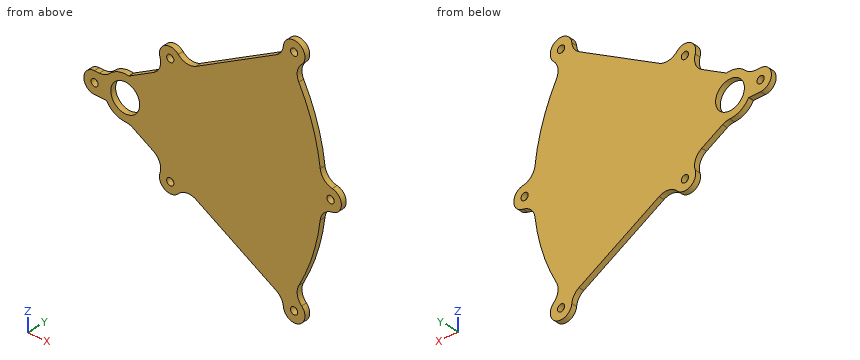
Autodesk Inventor part; units mm, degrees
ref_plane "YZ Plane" through (0, 0, 0) normal (1, 0, 0) x (0, 1, 0)
ref_plane "XZ Plane" through (0, 0, 0) normal (0, 1, 0) x (-1, 0, 0)
ref_plane "XY Plane" through (0, 0, 0) normal (0, 0, 1) x (1, 0, 0)
sketch "Sketch1" plane through (0, 0, 0) normal (0, 1, 0) x (-1, 0, 0)
  circle A0 centre (0, 0) radius 8
  arc A1 (-82.4777, 58.296) -> (-82.4777, -58.296) centre (0, 0) ccw construction
  arc A2 (-86.8253, 60.806) -> (-86.8253, -60.806) centre (0, 0) ccw construction
  arc A3 (-2, -11.8322) -> (-2, 11.8322) centre (0, 0) ccw
  line L0 (-2, -11.8322) -> (-89.433, -62.3116)
  arc A4 (-89.433, 62.3116) -> (-89.433, -62.3116) centre (0, 0) ccw
  line L1 (-2, 11.8322) -> (-89.433, 62.3116)
  circle A5 centre (-93.7631, -64.8116) radius 2
  circle A6 centre (-93.7631, 64.8116) radius 2
  circle A7 centre (-114, 0) radius 2
  circle A8 centre (-25, -30.8847) radius 2
  circle A9 centre (-25, 30.8847) radius 2
  circle A10 centre (17, 0) radius 2
  line L2 (10.3923, -6) -> (17, -6)
  arc A11 (17, -6) -> (17, 6) centre (17, 0) ccw
  line L3 (17, 6) -> (10.3923, 6)
  line L4 (-22.3038, -23.5546) -> (-19.8038, -27.8847)
  arc A12 (-30.1962, -33.8847) -> (-19.8038, -27.8847) centre (-25, -30.8847) ccw
  line L5 (-30.1962, -33.8847) -> (-32.6962, -29.5546)
  line L6 (-22.3038, 23.5546) -> (-19.8038, 27.8847)
  arc A13 (-19.8038, 27.8847) -> (-30.1962, 33.8847) centre (-25, 30.8847) ccw
  line L7 (-30.1962, 33.8847) -> (-32.6962, 29.5546)
  line L8 (-92.8025, 57.1726) -> (-96.9102, 59.7032)
  arc A14 (-88.567, 61.8116) -> (-96.9102, 59.7032) centre (-93.7631, 64.8116) ccw
  line L9 (-108.8347, -6) -> (-114, -6)
  arc A15 (-114, 6) -> (-114, -6) centre (-114, 0) ccw
  line L10 (-114, 6) -> (-108.8347, 6)
  line L11 (-92.8025, -57.1726) -> (-96.9102, -59.7032)
  arc A16 (-96.9102, -59.7032) -> (-88.567, -61.8116) centre (-93.7631, -64.8116) ccw
  point P0 (-109, 0)
  point P1 (12, 0)
  dimension "d0" = 16
  dimension "d1" = 101
  dimension "d3" = 12
  dimension "d6" = 60
  dimension "d7" = 2
  dimension "d8" = 5
  dimension "d9" = 3
  dimension "d10" = 4
  dimension "d12" = 5
  dimension "d13" = 5
  dimension "d14" = 5
  dimension "d15" = 5
  dimension "d16" = 5
  dimension "d17" = 5
  dimension "d18" = 25
  dimension "d19" = 6
  dimension "d20" = 6
extrude "Extrusion1" add sketch "Sketch1" along normal blind 3 contours L0 A4 L1 A3
extrude "Extrusion2" add sketch "Sketch1" along normal blind 3 contours A3 L3 A11 L2 | L4 A12 L5 L0 | A16 L11 A4 L0 | L1 L7 A13 L6 | L1 A4 L8 A14 | L9 A15 L10 A4
fillet "Fillet1" radius 8 12 edges at (32.6962, 1.5, 29.5546) (22.3038, 1.5, 23.5546) (88.567, 1.5, 61.8116) (92.8025, 1.5, 57.1726) (108.8347, 1.5, -6) (108.8347, 1.5, 6) (92.8025, 1.5, -57.1726) (88.567, 1.5, -61.8116) (32.6962, 1.5, -29.5546) (22.3038, 1.5, -23.5546) (2, 1.5, -11.8322) (-10.3923, 1.5, 6)
properties part number "RailBase" material "Polycarbonate, Clear"
Input: part model. Units: mm. Frame: model coordinates. Give positions to 0.01 mm unless a question says otherwise; leave off trailing zeros. Order: outer loops, then holes, each group sorted by start corner. A loop starts at its lowest first (then second) coordinate and runs counter-clockwise, first axis right, second up. Notation, with made-up numbers: (69, 63.5) - (126, 63.5) arc R35 cw to (126, 101.5) - close; hole circle Ø11 at (9, 86.5). An arc over 180 degrees is marked (long way). Answer as a JSON object with one key per item and string values. Group by question number.
Q1. Cut plane A-A, the plane z = 0. Output: boundary loops of the cut face in (x, y), then the cut area to 3 significant figures.
Q2. Line query: probe 1 along Z at (x, y) = (0, 2.1); probe 2 along X at (y, z) = (2.7, 1.5); probe 3 along Z at (x, y) = (-17, 2). Output: solid intervals per line, ascending.
Q3. Cut plane C-C, the plane x = -2. Output: boundary loops of the cut face in (y, z).
Q4. First-contact query: pin 1 Ø3.5 at (x, z) = (-17, 0) entering from +Y; pin 2 Ø1 at (x, z) = (69.5, -27.5) entering from -Y. Flat tips, straight axial feed; report the tip coordinate or a pass-through.
Q5. Cut plane D-D, the plane y = 1.95. Count the separate pieces of the cut face and the enclosed holes in it, then the cut area to 3 significant figures.
Q6. Cut plane B-B, the plane x = 25. Output: boundary loops of the cut face in (y, z).
Results:
{
 "1": {"outline": "(-23, 0) - (-19, 0) - (-19, 3) - (-23, 3) - close; (-15, 0) - (-8, 0) - (-8, 3) - (-15, 3) - close; (8, 0) - (112, 0) - (112, 3) - (8, 3) - close; (116, 0) - (120, 0) - (120, 3) - (116, 3) - close", "area": "357 mm^2"},
 "2": {"probe 1": "-12 to -8, 8 to 12", "probe 2": "-22.81 to -18.32, -15.68 to -7.86, 7.86 to 112.68, 115.32 to 119.81", "probe 3": "-6 to -2, 2 to 6"},
 "3": {"outline": "(0, -11.83) - (3, -11.83) - (3, -7.75) - (0, -7.75) - close; (0, 7.75) - (3, 7.75) - (3, 11.83) - (0, 11.83) - close"},
 "4": {"pin 1": "through", "pin 2": "y = 0"},
 "5": {"separate pieces": "1", "enclosed holes": "7", "area": "8,940 mm^2"},
 "6": {"outline": "(0, -36.88) - (3, -36.88) - (3, -32.88) - (0, -32.88) - close; (0, -28.88) - (3, -28.88) - (3, 28.88) - (0, 28.88) - close; (0, 32.88) - (3, 32.88) - (3, 36.88) - (0, 36.88) - close"}
}
